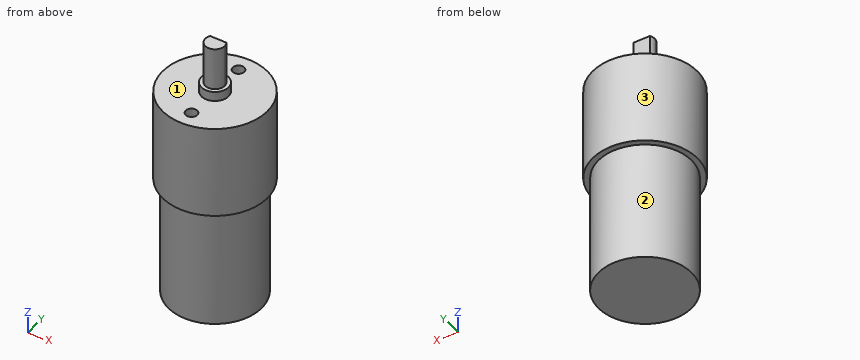
```python
from build123d import *

# Parameters (mm, degrees)
SKETCH1_R           = 13.5
BOSS_EXTRUDE1_DEPTH = 24
BOSS_EXTRUDE2_START = -24
SKETCH1_3_R         = 12
BOSS_EXTRUDE2_DEPTH = 31
SKETCH2_R           = 3.5
BOSS_EXTRUDE3_DEPTH = 2.5
BOSS_EXTRUDE4_START = 2.5
BOSS_EXTRUDE4_DEPTH = 11
SKETCH3_R           = 1.5
CUT_EXTRUDE1_DEPTH  = 4


with BuildPart() as part:
    # Sketch1 → Boss-Extrude1 (new body)
    with BuildSketch(Plane.XY):
        Circle(SKETCH1_R)
    extrude(amount=-BOSS_EXTRUDE1_DEPTH)

    # Sketch1<3> → Boss-Extrude2 (add)
    with BuildSketch(Plane.XY.offset(BOSS_EXTRUDE2_START)):
        Circle(SKETCH1_3_R)
    extrude(amount=-BOSS_EXTRUDE2_DEPTH)

    # Sketch2 → Boss-Extrude3 (add)
    with BuildSketch(Plane.XY):
        Circle(SKETCH2_R)
    extrude(amount=BOSS_EXTRUDE3_DEPTH)

    # Sketch2<3> → Boss-Extrude4 (add)
    with BuildSketch(Plane.XY.offset(BOSS_EXTRUDE4_START)):
        with BuildLine():
            Line((2.13541565, 1.3), (-2.13541565, 1.3))
            ThreePointArc((-2.13541565, 1.3), (-0.675078097, -2.407128905), (2.5, 0))
            ThreePointArc((2.5, 0), (2.407128905, 0.675078097), (2.13541565, 1.3))
        make_face()
    extrude(amount=BOSS_EXTRUDE4_DEPTH)

    # Sketch3 → Cut-Extrude1 (cut)
    with BuildSketch(Plane.XY):
        with Locations((0, 9.25)):
            Circle(SKETCH3_R)
        with Locations((0, -9.25)):
            Circle(SKETCH3_R)
    extrude(amount=-CUT_EXTRUDE1_DEPTH, mode=Mode.SUBTRACT)


solid = part.part
```
Geometry: final body of the model. Coordinates: model frame, mm. Face numbers are marked on the shaded views. A direction names the side the tool comes from. Round coordinates to 2 decimals unless told otherwise and drop trailing zeros. Order: outer loops, then holes, each group sorted by start corner. A loop starts at its lowest first (then second) coordinate and runs counter-clockwise, first axis right, second up. Notation, with made-up numbers: (41, 5.25) -> (68, 5.25) arc R14 ccw to (68, 14.25) -> close; hole circle Ø5 at (16.5, 29.5). An arc over 180 degrees is marked (long way). Use one line per item in the form item = value.
(1) Section D-D on z = -32.5. Return loops of the section in (x, y).
Results list:
outline = circle Ø24 at (0, 0)
(2) Section A-A on x = 0. Return loops of the section in (y, z), and give its area (3 significant figures).
Results list:
outline = (-13.5, -24) -> (-12, -24) -> (-12, -55) -> (12, -55) -> (12, -24) -> (13.5, -24) -> (13.5, 0) -> (10.75, 0) -> (10.75, -4) -> (7.75, -4) -> (7.75, 0) -> (3.5, 0) -> (3.5, 2.5) -> (1.3, 2.5) -> (1.3, 13.5) -> (-2.5, 13.5) -> (-2.5, 2.5) -> (-3.5, 2.5) -> (-3.5, 0) -> (-7.75, 0) -> (-7.75, -4) -> (-10.75, -4) -> (-10.75, 0) -> (-13.5, 0) -> close
area = 1,430 mm^2
(3) Ray query, probe 1 along Y at (x, z) = (0, -1.35); probe 2 along Y at (x, z) = (1.25, -1); probe 3 along Y at (x, z) = (-0.5, -17). Return the intervals inside material, ascending. Write a range as [from, to].
Results list:
probe_1 = [-13.5, -10.75], [-7.75, 7.75], [10.75, 13.5]
probe_2 = [-13.44, -10.08], [-8.42, 8.42], [10.08, 13.44]
probe_3 = [-13.49, 13.49]
(4) Access query for the marked faces 1, 2 and 3. Directions: +Z, -Z, +X, -X, +Y, -Y. A direction counts if a zero-diameter tool reaches every point of the face in a straight line with its end or side. Return the directions, or none.
Results list:
face_1 = +Z
face_2 = -Z
face_3 = +Z, -Z
(5) First-contact query: pin 1 Ø8 at (y, z) = (6.5, 6) entering from +X; pin 2 Ø8 at (x, z) = (0, 4.5) entering from -Y; pin 3 Ø1.5 at (x, y) = (0.5, -9.5) entering from +Z; pin 4 Ø6 at (x, y) = (7, 3.5) entering from +Z. Flat tips, straight axial feed; report the tip coordinate or a pass-through.
Results list:
pin_1 = through
pin_2 = -3.5
pin_3 = -4
pin_4 = 0
(6) Section C-C on z = -3. Return loops of the section in (x, y), and give its area (3 significant figures).
Results list:
outline = circle Ø27 at (0, 0); hole circle Ø3 at (0, -9.25); hole circle Ø3 at (0, 9.25)
area = 558 mm^2
(7) Section B-B on y = 5. Return loops of the section in (x, z), and give its area (3 significant figures).
Results list:
outline = (-12.54, -24) -> (-10.91, -24) -> (-10.91, -55) -> (10.91, -55) -> (10.91, -24) -> (12.54, -24) -> (12.54, 0) -> (-12.54, 0) -> close
area = 1,280 mm^2
